from build123d import *

# Parameters (mm, degrees)
SKETCH_1_R      = 2.75
EXTRUDE_1_DEPTH = 5


with BuildPart() as part:
    # 草圖1 → 填料-伸長1 (new body)
    with BuildSketch(Plane.XY):
        with BuildLine():
            Line((17, 7), (30, 7))
            ThreePointArc((30, 7), (37, 0), (30, -7))
            Line((30, -7), (-2, -7))
            ThreePointArc((-2, -7), (-5.535533906, -5.535533906), (-7, -2))
            Line((-7, -2), (-7, 32.95836944))
            ThreePointArc((-7, 32.95836944), (-7.761204675, 36.785203763), (-9.928932188, 40.029437252))
            Line((-9.928932188, 40.029437252), (-12.02081528, 42.121320344))
            ThreePointArc((-12.02081528, 42.121320344), (-12.02081528, 52.02081528), (-2.121320344, 52.02081528))
            Line((-2.121320344, 52.02081528), (4.071067812, 45.828427125))
            ThreePointArc((4.071067812, 45.828427125), (6.238795325, 42.584193637), (7, 38.757359313))
            Line((7, 38.757359313), (7, 17))
            ThreePointArc((7, 17), (9.928932188, 9.928932188), (17, 7))
        make_face()
        Circle(SKETCH_1_R, mode=Mode.SUBTRACT)
        with Locations((30, 0)):
            Circle(SKETCH_1_R, mode=Mode.SUBTRACT)
        with Locations((-7.071067812, 47.071067812)):
            Circle(SKETCH_1_R, mode=Mode.SUBTRACT)
    extrude(amount=EXTRUDE_1_DEPTH)


solid = part.part
Verification items for the finished model (mm, model axes). A direction names the side the tool comes from. Coordinates: 2 decimals unless noted, no trailing zeros. Order: outer loops, then holes, each group sorted by start corner. A loop starts at its lowest first (then second) coordinate and runs counter-clockwise, first axis right, second up. Notation, with made-up numbers: (-22, 41) -> (-11, 41) arc R27 ccw to (-11, 74) -> close; hole circle Ø2 at (-4.5, 27). An arc over 180 degrees is marked (long way). Use CSV: the item, a comma, the result in double quotes. Start each with the question number.
Q1. Depth check by flat-ended pin: P1, Ø1, axis at x = 28.5, z = 3, coming from the +Y side; P2, Ø1, axis at x = 16, z = 3, coming from the +Y side; P3, Ø1.5, axis at y = 29, z = 2.5, coming from the +X side. Enter the tip coordinate at first touch or a pass-through.
Q2. Section check A-A, the plane y = 0. Record the cut outline in (x, z), and give its area (3 significant figures).
Q3. Section check C-C, the plane z = 3.1. Record the cut outline in (x, y), and give its area (3 significant figures).
Q4. Tool access check on faces 5 (the flat face through (23, 7, 2)), 6 (the flat face through (14, -7, 2)). Record the directions out of +Z, -Z, +X, -X, +Y, -Y that give a thin tool (end or side, any length) a straight path to the whole face; none if there is none.
Q5. Thickness scan on line 1 along X through (y, z) = (-2.5, 3.35); line 2 along X through (y, z) = (-1, 1.35); line 3 along Y through (x, z) = (0, 2.35). Record the ranges inside material, lowest first.
Q6. Section check D-D, the plane y = 18.5. Record the cut outline in (x, z), and give its area (3 significant figures).
Q7. Section check B-B, the plane x = 0. Record the cut outline in (y, z).
Q8. Draft check along Y on faces 1 (the cylindrical face through (9.85, 10.01, 2.46)), 2 (the flat face through (-7, 15, 2)), 3 (the cylindrical face through (-12.13, 51.91, 2.46)), 4 (the cylindrical face through (-0.596, -2.685, 2.465)). Enter one of: +Y half, -Y half, draft (parallel to the pull), parting line (faces both ways), or undercut.
Returned:
1,P1,"stops at y = 7"
1,P2,"stops at y = 7.11"
1,P3,"stops at x = 7"
2,outline,"(-7, 0) -> (-2.75, 0) -> (-2.75, 5) -> (-7, 5) -> close; (2.75, 0) -> (27.25, 0) -> (27.25, 5) -> (2.75, 5) -> close; (32.75, 0) -> (37, 0) -> (37, 5) -> (32.75, 5) -> close"
2,area,"165 mm^2"
3,outline,"(-12.02, 42.12) -> (-9.93, 40.03) arc R10 cw to (-7, 32.96) -> (-7, -2) arc R5 ccw to (-2, -7) -> (30, -7) arc R7 ccw to (30, 7) -> (17, 7) arc R10 cw to (7, 17) -> (7, 38.76) arc R10 ccw to (4.07, 45.83) -> (-2.12, 52.02) arc R7 ccw to start; hole circle Ø5.5 at (-7.07, 47.07); hole circle Ø5.5 at (0, 0); hole circle Ø5.5 at (30, 0)"
3,area,"1,220 mm^2"
4,face 5,"+Z, -Z, +X, +Y"
4,face 6,"+Z, -Z, +X, -X, -Y"
5,line 1,"x = -6.97 to -1.15, 1.15 to 28.85, 31.15 to 36.54"
5,line 2,"x = -7 to -2.56, 2.56 to 27.44, 32.56 to 36.93"
5,line 3,"y = -7 to -2.75, 2.75 to 49.9"
6,outline,"(-7, 0) -> (7, 0) -> (7, 5) -> (-7, 5) -> close"
6,area,"70.0 mm^2"
7,outline,"(-7, 0) -> (-2.75, 0) -> (-2.75, 5) -> (-7, 5) -> close; (2.75, 0) -> (49.9, 0) -> (49.9, 5) -> (2.75, 5) -> close"
8,face 1,"+Y half"
8,face 2,"draft"
8,face 3,"parting line"
8,face 4,"undercut"
